The drawing under review shows one solid part. Ordinate dimensions are in mm from its lowest x, y, z. Coordinates: 2 decimals unless noted, no trailing zeros. Order: outer loops, then holes, each group sorted by start corner. A loop starts at its lowest first (then second) coordinate and runs counter-clockwise, first axis right, second up. Notation, with made-up numbers: (69, 40) - (100, 40) arc R19 cw to (100, 45) - close; hole circle Ø4 at (-31.5, 29). An arc over 180 degrees is marked (long way). Answer in a Markdown table with one row per item.
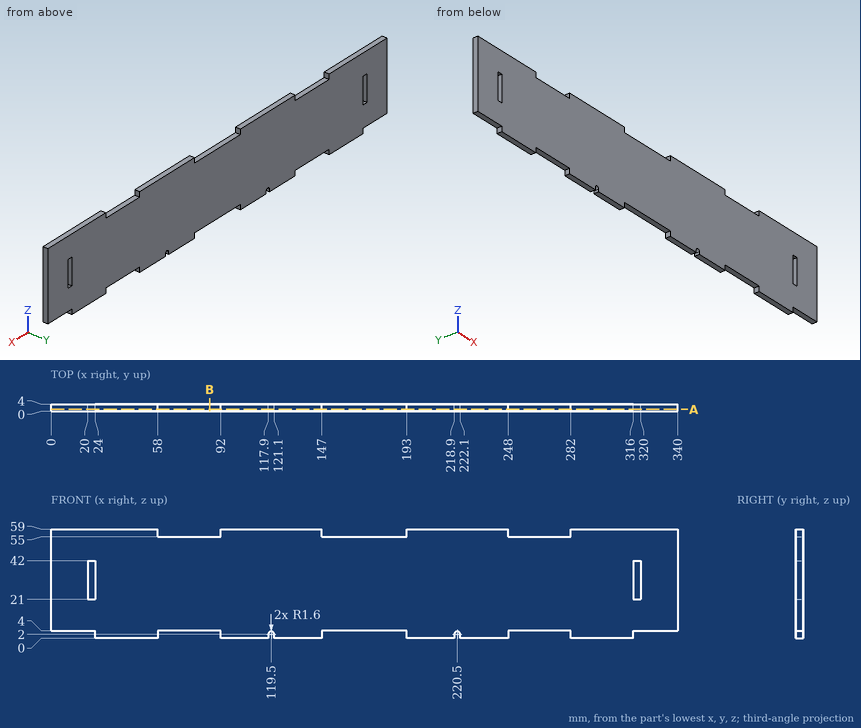
Item 1: To check wall thickness, follow line 1 (X direction, y = 3.7, z = 39); line 2 (Z direction, x = 252, y = 2.1). State the ranges of each line that lie inside material, in increasing order. Write a range as from..to.
Check values:
| item | result |
|---|---|
| line 1 | 0..20, 24..316, 320..340 |
| line 2 | 4..55 |
Item 2: Clearance check with flat-ended pins moving along their axes: pin 1 Ø1.2 at (x, y) = (21.5, 2) entering from -Z; pin 2 Ø1.2 at (y, z) = (3, 1) entering from -X; pin 3 Ø2 at (y, z) = (2, 1.5) entering from +X. State where each tip first meets the part, or that it passes through.
Check values:
| item | result |
|---|---|
| pin 1 | z = 4 |
| pin 2 | x = 24 |
| pin 3 | x = 316 |
Item 3: We need section A-A, the plane y = 1.05. State how many separate pieces and enclosed holes the cut face has, then the cut area to 3 significant figures.
Check values:
| item | result |
|---|---|
| separate pieces | 1 |
| enclosed holes | 2 |
| area | 18,800 mm^2 |
Item 4: We need section B-B, the plane x = 86. Write out the cut boundary in (y, z).
Check values:
| item | result |
|---|---|
| outline | (0, 4) - (4, 4) - (4, 55) - (0, 55) - close |
